Autodesk Inventor part; units mm, degrees
ref_plane "YZ Plane" through (0, 0, 0) normal (1, 0, 0) x (0, 1, 0)
ref_plane "XZ Plane" through (0, 0, 0) normal (0, 1, 0) x (-1, 0, 0)
ref_plane "XY Plane" through (0, 0, 0) normal (0, 0, 1) x (1, 0, 0)
sketch "草圖1" plane through (0, 0, 0) normal (0, 1, 0) x (-1, 0, 0)
  line L0 (0, 0) -> (-60, 0)
  line L1 (-60, 0) -> (-60, -40)
  line L2 (-60, -40) -> (0, -40)
  line L3 (0, -40) -> (0, 0)
  dimension "d0" = 40
  dimension "d1" = 60
extrude "擠出1" add sketch "草圖1" along normal blind 10
sketch "草圖2" plane through (0, 0, 0) normal (0, 0, 1) x (1, 0, 0)
  line L0 (0, 10) -> (60, 10)
  line L1 (0, 10) -> (30, 10)
  line L2 (30, 10) -> (30, 20)
  line L3 (30, 20) -> (0, 20)
  line L4 (0, 20) -> (0, 10)
  point P0 (0, 0)
  dimension "d4" = 30
  dimension "d5" = 10
extrude "擠出2" add sketch "草圖2" against normal blind 10
sketch "草圖3" plane through (60, 0, -40) normal (0, 0, -1) x (-1, 0, 0)
  line L0 (0, 10) -> (60, 10)
  line L1 (0, 10) -> (30, 10)
  line L2 (30, 10) -> (30, 40)
  line L3 (30, 40) -> (0, 40)
  line L4 (0, 40) -> (0, 10)
  line L5 (60, 0) -> (60, 10)
  line L6 (30, 40) -> (60, 10)
  line L7 (10, 30) -> (20, 30)
  line L8 (20, 30) -> (20, 20)
  line L9 (20, 20) -> (10, 20)
  line L10 (10, 20) -> (10, 30)
  dimension "d8" = 30
  dimension "d9" = 30
  dimension "d10" = 10
extrude "擠出3" add sketch "草圖3" against normal blind 10
chamfer "倒角1" distance 20 angle 45 1 edges at (60, 5, 0)
properties part number "12"
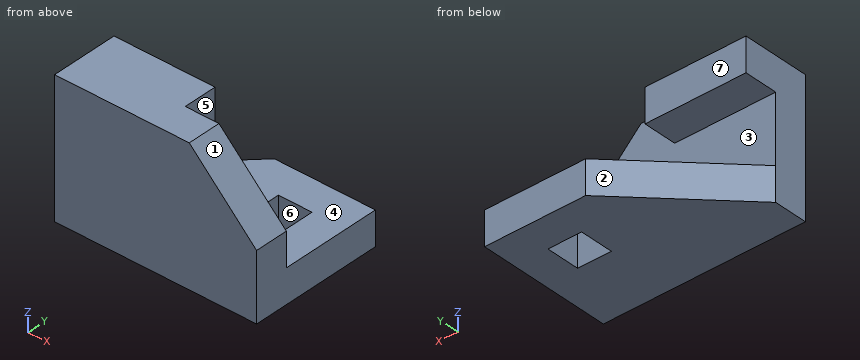
Could you check a few things on this model? Use its own coordinates, in mm. Face numbers are marked on the shaded views. A direction names the side the tool comes from. Coordinates: 2 decimals unless noted, no trailing zeros. Loops run counter-clockwise (first coordinate to the right, second up) from the corner with the lowest first, then second, coordinate; pieces in that order, holes last.
1. For P1, Ø3, axis at y = 16, z = -5, coming from the +X side; P2, Ø5, axis at x = 15.5, z = -6.5, coming from the +Y side; P3, Ø8, axis at x = 53, y = 9, coming from the +Z side; P4, Ø12, axis at y = 18, z = -18, coming from the +X side, each with a flat end and sliding along its axis, tell me the tip position at first contact or that it passes through.
2. Imagine slicing it at A-A (y = 23.5). Please give me the cut outline in (x, z), and give its area (3 significant figures).
3. For the marked faces 4, 5, 6 and 7, which set-ups out of +Z, -Z, +X, -X, +Y, -Y let a thin tool reach every point of the face, with its end or its side?
4. Imagine slicing it at B-B (z = -37). Please give me the cut outline in (x, y).
5. Imagine slicing it at C-C (x = 10). Please give me the cut outline in (y, z), and give its area (3 significant figures).
6. I need wall thicknesses on L1, parallel to Z at x = 53.5, y = 23; L2, parallel to Y at x = 4, z = -27; L3, parallel to X at y = 19, z = -1.5. Which ranges of each line are inside material? Lowest first, please.
7. Imagine slicing it at D-D (z = -9). Please give me the cut outline in (x, y).
8. We'd pull the mould along Z, two halves only. Please class the marked faces 1, 2 and 3: released by +Z, released by -Z, zero draft, split by the parting line, or undercut.
Computed values:
1. P1: stops at x = 30
1. P2: stops at y = 20
1. P3: stops at z = -9
1. P4: passes through
2. outline: (13.5, -40) - (40, -40) - (40, -30) - (13.5, -30) - close; (50, -40) - (60, -40) - (60, -30) - (50, -30) - close
2. area: 365 mm2
3. face 4: +X, -X, +Y
3. face 5: +Z, +X, +Y
3. face 6: +Z, -Z
3. face 7: +Z, +X, -X, +Y
4. outline: (0, 0) - (60, 0) - (60, 40) - (30, 40) - (0, 10) - close; hole (40, 20) - (50, 20) - (50, 30) - (40, 30) - close
5. outline: (0, -40) - (20, -40) - (20, -30) - (10, -30) - (10, -10) - (20, -10) - (20, 0) - (0, 0) - close
5. area: 600 mm2
6. L1: z = -40 to -30
6. L2: y = 0 to 10
6. L3: x = 0 to 30
7. outline: (0, 0) - (49, 0) - (49, 10) - (30, 10) - (30, 20) - (0, 20) - close
8. face 1: released by +Z
8. face 2: zero draft
8. face 3: undercut
